from build123d import *

# Parameters (mm, degrees)
ESQUISSE1_W        = 30
ESQUISSE1_H        = 30
BOSS_EXTRU_1_DEPTH = 3
BOSS_EXTRU_2_DEPTH = 2.5


with BuildPart() as part:
    # Esquisse1 → Boss.-Extru.1 (new body)
    with BuildSketch(Plane.XY):
        with Locations((15, -15)):
            Rectangle(ESQUISSE1_W, ESQUISSE1_H)
    extrude(amount=BOSS_EXTRU_1_DEPTH)

    # Esquisse4 → Boss.-Extru.2 (add, symmetric)
    with BuildSketch(Plane.ZY.offset(-15)):
        with BuildLine():
            Line((0, -12.173324278), (0, -13.673324278))
            ThreePointArc((0, -13.673324278), (-5.548147475, -15.256657612), (0, -16.839990945))
            Line((0, -16.839990945), (0, -18.339990945))
            ThreePointArc((0, -18.339990945), (-6.548147475, -15.256657612), (0, -12.173324278))
        make_face()
    extrude(amount=BOSS_EXTRU_2_DEPTH, both=True)


solid = part.part
Design review of the part built by this model. Coordinates are the model's own, in mm. A direction names the side the tool comes from. Coordinates: 2 decimals unless noted, no trailing zeros. Order: outer loops, then holes, each group sorted by start corner. A loop starts at its lowest first (then second) coordinate and runs counter-clockwise, first axis right, second up.
Item 1: Take a section at A-A, the plane z = -0.75. Write out the cut boundary in (x, y), then the cut area to 3 significant figures.
Item 2: For line 1 (Z direction, x = 14.5, y = -12.5); line 2 (Y direction, x = 14.5, z = -0.75); line 3 (Z direction, x = 24.25, y = -1.5), list the stretches that pass through material, from the lowest coordinate up.
Item 3: The part is to be moulded in two halves that separate along Z. For faces 1 (the cylindrical face through (14.965, -15.148, -5.546)), 2 (the flat face through (17.5, -15, -6)), 3 (the flat face through (15, -15, 3)), 4 (the cylindrical face through (14.965, -15.383, -6.546)), say which applies: pulls with the +Z half, pulls with the -Z half, needs draft (parallel to the pull), parting line crosses it, or undercut.
Item 4: Take a section at C-C, the plane x = 26.25. Write out the cut boundary in (y, z), then the cut area to 3 significant figures.
Item 5: For faces 5 (the flat face through (12.5, -15, -6)), 6 (the flat face through (30, -15, 1)), list the 3-axis set-ups (+Z, -Z, +X, -X, +Y, -Y) from which the entire face can be reached by the end or side of a thin tool; tool diameter is ignored.
Item 6: Take a section at B-B, the plane y = -14.5. Write out the cut boundary in (x, z).
Item 7: For pin 1 Ø1 at (y, z) = (-26.5, -1) entering from -X; pin 2 Ø5 at (y, z) = (-17, -5) entering from -X; pin 3 Ø1 at (x, y) = (5.5, -4.5) entering from -Z, all flat-tipped, find the tip position at first contact; note any pin that passes through.
Item 8: Take a section at D-D, the plane y = -9.75. Write out the cut boundary in (x, z), then the cut area to 3 significant figures.
The answers:
1. outline: (12.5, -18.83) - (17.5, -18.83) - (17.5, -17.66) - (12.5, -17.66) - close; (12.5, -12.86) - (17.5, -12.86) - (17.5, -11.68) - (12.5, -11.68) - close
1. area: 11.7 mm2
2. line 1: z = -5.45 to -3.73, -1.36 to 3
2. line 2: y = -18.83 to -17.66, -12.86 to -11.68
2. line 3: z = 0 to 3
3. face 1: undercut
3. face 2: needs draft
3. face 3: pulls with the +Z half
3. face 4: undercut
4. outline: (-30, 0) - (0, 0) - (0, 3) - (-30, 3) - close
4. area: 90.0 mm2
5. face 5: -Z, -X, +Y, -Y
5. face 6: +Z, -Z, +X, +Y, -Y
6. outline: (0, 0) - (30, 0) - (30, 3) - (0, 3) - close; (12.5, -6.48) - (17.5, -6.48) - (17.5, -5.45) - (12.5, -5.45) - close
7. pin 1: passes through
7. pin 2: stops at x = 12.5
7. pin 3: stops at z = 0
8. outline: (0, 0) - (30, 0) - (30, 3) - (0, 3) - close
8. area: 90.0 mm2
